Input: dimensioned drawing with shaded views. Units: mm. Origin: part minimum x, y, z. Give positions to 0.01 mm unless a question says otherwise; leave off trailing zeros. Loops run counter-clockwise (first coordinate to the right, second up) from the corner with the lowest first, then second, coordinate; pieces in that order, holes last. Notation, with made-up numbers: (22.25, -6.5) -> (74.25, -6.5) arc R30 ccw to (74.25, 18.5) -> close; hole circle Ø10 at (-30, -36.5). An arc over 180 degrees is marked (long way). Answer in a Markdown table with one row per item. Add a question column.
1) First-contact query: P1, Ø9, axis at x = 80, y = 96, coming from the -Z side. Flat tip, straight axial feed; report the tip coordinate or a pass-through.
2) Line query: line 1 (X direction, y = 96, z = 2); line 2 (Y direction, x = 150.1, z = 1.4); line 3 (X direction, y = 51, z = 0.5). Output: solid intervals per line, ascending. Write a range as from..to.
3) Section query D-D (x = 43). Return the cut outline in (y, z), plus the area to 3 significant figures.
4) Section query A-A (y = 34). Return the cut outline in (x, z).
5) Section query C-C (y = 96). Return the cut outline in (x, z), plus the area to 3 significant figures.
6) Section query B-B (x = 150.1). Return the cut outline in (y, z), plus the area to 3 significant figures.
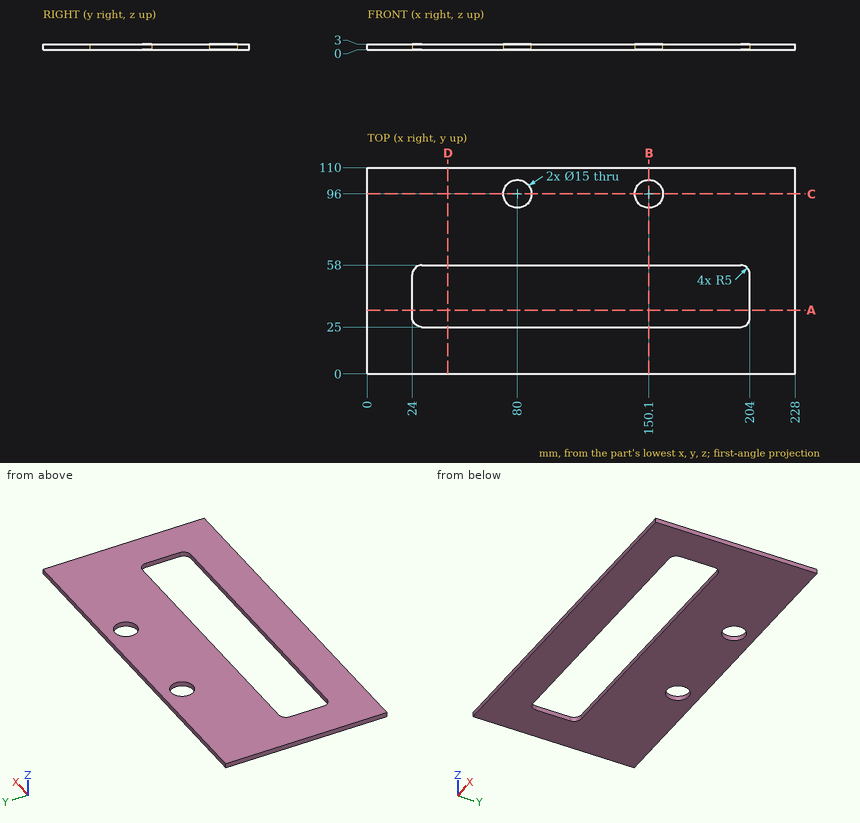
Evaluation:
| question | item | result |
|---|---|---|
| 1 | P1 | through |
| 2 | line 1 | 0..72.5, 87.5..142.6, 157.6..228 |
| 2 | line 2 | 0..25, 58..88.5, 103.5..110 |
| 2 | line 3 | 0..24, 204..228 |
| 3 | outline | (0, 0) -> (25, 0) -> (25, 3) -> (0, 3) -> close; (58, 0) -> (110, 0) -> (110, 3) -> (58, 3) -> close |
| 3 | area | 231 mm² |
| 4 | outline | (0, 0) -> (24, 0) -> (24, 3) -> (0, 3) -> close; (204, 0) -> (228, 0) -> (228, 3) -> (204, 3) -> close |
| 5 | outline | (0, 0) -> (72.5, 0) -> (72.5, 3) -> (0, 3) -> close; (87.5, 0) -> (142.6, 0) -> (142.6, 3) -> (87.5, 3) -> close; (157.6, 0) -> (228, 0) -> (228, 3) -> (157.6, 3) -> close |
| 5 | area | 594 mm² |
| 6 | outline | (0, 0) -> (25, 0) -> (25, 3) -> (0, 3) -> close; (58, 0) -> (88.5, 0) -> (88.5, 3) -> (58, 3) -> close; (103.5, 0) -> (110, 0) -> (110, 3) -> (103.5, 3) -> close |
| 6 | area | 186 mm² |
